The drawing under review shows one solid part. Ordinate dimensions are in mm from its lowest x, y, z. A direction names the side the tool comes from. Round coordinates to 2 decimals unless told otherwise and drop trailing zeros. Write each loop counter-clockwise with the first axis right and the second up, starting at its lowest first coordinate (ties: lowest second). Pieces come first, ordered by that corner, then holes. Notation, with made-up numbers: (-20, -18) - (-2, -18) arc R23 ccw to (-2, -7) - close; hole circle Ø4 at (39, -7). An arc over 180 degrees is marked (long way). Answer in a Markdown table with one row per item. Add a question column.
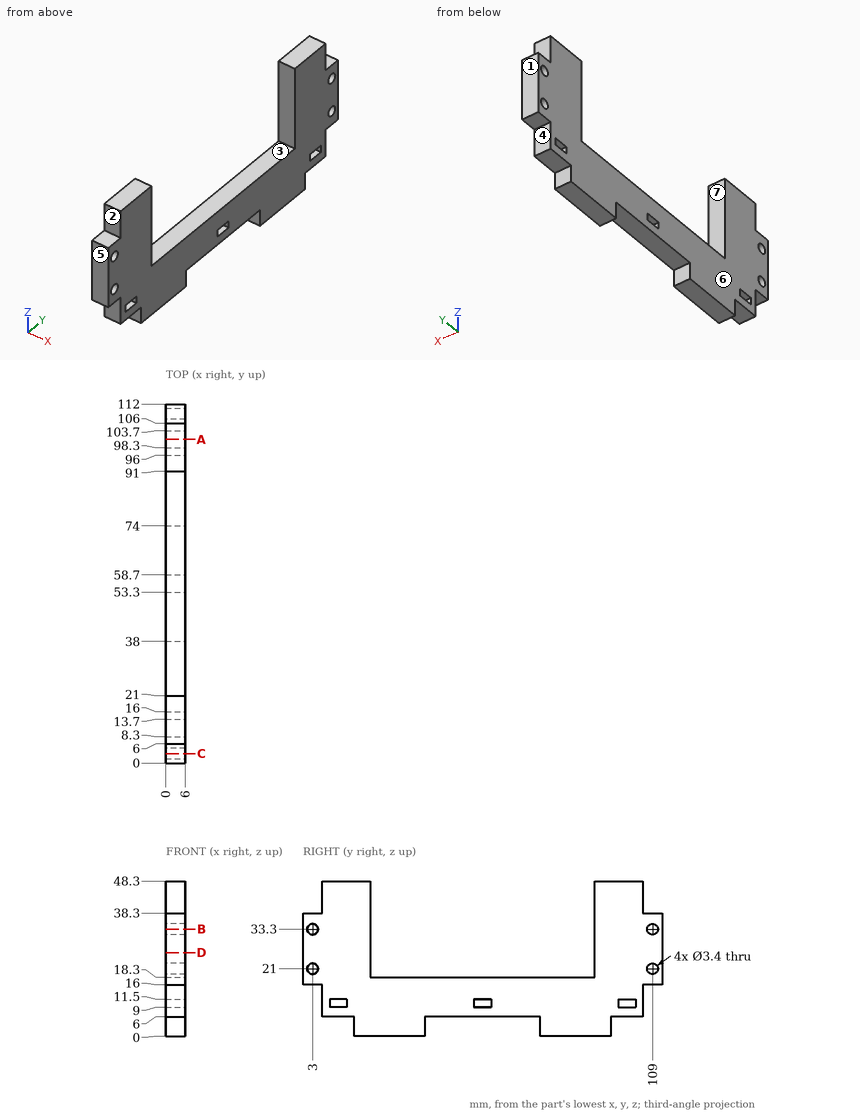
Q1. Insertion check: pin 1 Ø3 at (x, z) = (4, 33.5) entering from -Y; pin 2 Ø0.8 at (x, z) = (2, 10.5) entering from -Y; pin 3 Ø3 at (x, z) = (1.5, 4) entering from -Y; pin 4 Ø3 at (x, z) = (2, 10) entering from +Y. Each pin has a flat end and moves straight along its axis. Give the tip position at first contact, or say it passes through.
Q2. Add section A-A on y = 101. State the section outline as (x, z) points.
Q3. Add section C-C on y = 3. State the section outline as (x, z) points, then the cut area to 3 significant figures.
Q4. To check wall thickness, follow probe 1 along Y at (x, z) = (2.45, 10); probe 2 along Y at (x, z) = (1.3, 21); probe 3 along Z at (x, y) = (1.7, 3). State the ranges of each line that lie inside material, in increasing order.
Q5. Add section B-B on z = 33.3. State the section outline as (x, y) points, then the cut area to 3 significant figures.
Q6. Add section D-D on z = 26. State the section outline as (x, y) points, then the cut area to 3 significant figures.
Q7. Tool access review of the marked faces 1, 2 and 3: name each direction out of +Z, -Z, +X, -X, +Y, -Y from which nothing blocks a thin tool from reaching the whole face with its end or side.
Q8. Draft analysis for pull direction Y (two halves, no side actions). For the marked faces 4, 5, 6 and 7, state which applies: released by +Y, released by -Y, zero draft, split by the parting line, or undercut.
Answer sheet:
| question | item | result |
|---|---|---|
| 1 | pin 1 | stops at y = 0 |
| 1 | pin 2 | stops at y = 6 |
| 1 | pin 3 | stops at y = 16 |
| 1 | pin 4 | stops at y = 106 |
| 2 | outline | (0, 6) - (6, 6) - (6, 9) - (0, 9) - close; (0, 11.5) - (6, 11.5) - (6, 48.3) - (0, 48.3) - close |
| 3 | outline | (0, 16) - (6, 16) - (6, 19.3) - (0, 19.3) - close; (0, 22.7) - (6, 22.7) - (6, 31.6) - (0, 31.6) - close; (0, 35) - (6, 35) - (6, 38.3) - (0, 38.3) - close |
| 3 | area | 93.0 mm² |
| 4 | probe 1 | y = 6 to 8.3, 13.7 to 53.3, 58.7 to 98.3, 103.7 to 106 |
| 4 | probe 2 | y = 0 to 1.3, 4.7 to 21, 91 to 107.3, 110.7 to 112 |
| 4 | probe 3 | z = 16 to 19.3, 22.7 to 31.6, 35 to 38.3 |
| 5 | outline | (0, 0) - (6, 0) - (6, 1.3) - (0, 1.3) - close; (0, 4.7) - (6, 4.7) - (6, 21) - (0, 21) - close; (0, 91) - (6, 91) - (6, 107.3) - (0, 107.3) - close; (0, 110.7) - (6, 110.7) - (6, 112) - (0, 112) - close |
| 5 | area | 211 mm² |
| 6 | outline | (0, 0) - (6, 0) - (6, 21) - (0, 21) - close; (0, 91) - (6, 91) - (6, 112) - (0, 112) - close |
| 6 | area | 252 mm² |
| 7 | face 1 | +Z, -Z, +X, -X, +Y |
| 7 | face 2 | +Z, +X, -X, -Y |
| 7 | face 3 | +Z, +X, -X |
| 8 | face 4 | released by +Y |
| 8 | face 5 | released by -Y |
| 8 | face 6 | zero draft |
| 8 | face 7 | undercut |
